from build123d import *

# Parameters (mm, degrees)
BOSS_EXTRUDE1_DEPTH = 20
BOSS_EXTRUDE2_DEPTH = 40
SKETCH1_4_W         = 15
SKETCH1_4_H         = 20
BOSS_EXTRUDE3_DEPTH = 20


with BuildPart() as part:
    # Sketch1 → Boss-Extrude1 (new body)
    with BuildSketch(Plane(origin=(0, 0, 0), x_dir=(1, 0, 0), z_dir=(0, 1, 0))):
        Polygon((20, -30), (0, -30), (0, -50), (15, -100), (22.5, -100), (22.5, -70), (35, -70), (35, -30), align=None)
        Polygon((50, -30), (35, -30), (35, -70), (47.5, -70), (47.5, -100), (55, -100), (70, -50), (70, -30), align=None)
    extrude(amount=BOSS_EXTRUDE1_DEPTH)

    # Sketch1_3 → Boss-Extrude2 (add)
    with BuildSketch(Plane(origin=(0, 0, 0), x_dir=(1, 0, 0), z_dir=(0, 1, 0))):
        Polygon((0, -30), (0, 0), (15, 0), (15, -10), (20, -10), (20, -30), align=None)
        Polygon((70, -30), (70, 0), (55, 0), (55, -10), (50, -10), (50, -30), align=None)
    extrude(amount=BOSS_EXTRUDE2_DEPTH)

    # Sketch1_4 → Boss-Extrude3 (add)
    with BuildSketch(Plane(origin=(0, 0, 0), x_dir=(1, 0, 0), z_dir=(0, 1, 0))):
        with Locations((27.5, -20)):
            Rectangle(SKETCH1_4_W, SKETCH1_4_H)
        with Locations((42.5, -20)):
            Rectangle(SKETCH1_4_W, SKETCH1_4_H)
    extrude(amount=BOSS_EXTRUDE3_DEPTH)


solid = part.part
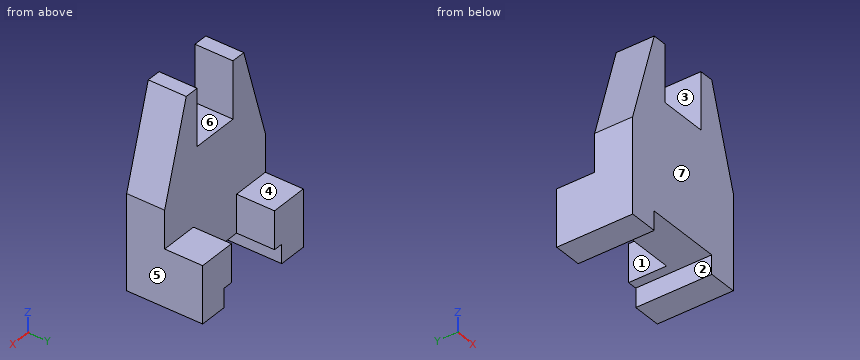
Here's how the part is built. I have some questions about the finished solid (model axes, mm). Face numbers are marked on the shaded views. A direction names the side the tool comes from. Give positions to 0.01 mm unless a question says otherwise; leave off trailing zeros. Write each loop counter-clockwise with the first axis right and the second up, starting at its lowest first coordinate (ties: lowest second). Pieces come first, ordered by that corner, then holes. Notation, with made-up numbers: (-7, 71) -> (4, 71) arc R12 cw to (4, 93) -> close; hole circle Ø1 at (17, 4.5). An arc over 180 degrees is marked (long way). Use one line per item in the form item = value. Start each with the question number.
1. Imagine slicing it at C-C on y = 4.5. List the corners of the cut face in (x, z) for me, plus the area to 3 significant figures.
2. Imagine slicing it at A-A on y = 22.5. List the corners of the cut face in (x, z) for me.
3. Thinking about a two-plate mould opening in X: for the marked faces 5, 6 and 7, which applies, +X half, -X half, draft (parallel to the pull), parting line (faces both ways), or undercut?
4. Will these pins go through, and if not, where does the flat tip stop? pin 1 Ø1 at (x, z) = (11, 40.5) entering from +Y; pin 2 Ø16 at (y, z) = (13, 83.5) entering from -X; pin 3 Ø10 at (y, z) = (6.5, 85) entering from +X.
5. If I drill on L1, parallel to Y at x = 13, z = 85.5; L2, parallel to Z at x = 6.5, y = 27; L3, parallel to X at y = 16, z = 87.5, over which ranges is the centre line in solid material (lowest first)?
6. Imagine slicing it at D-D on x = 10.5. List the corners of the cut face in (y, z) for me, plus the area to 3 significant figures.
7. On a 3-axis mill with a long thin cutter (end or side, diameter ignored), from which of +Z, -Z, +X, -X, +Y, -Y can I reach the whole of each face in a straight line? I mean the marked faces 1, 2, 3 and 4. Say none if no direction works.
8. Imagine slicing it at B-B on z = 83.5. List the corners of the cut face in (x, y) for me, plus the area to 3 significant figures.
Entries:
q1.outline = (0, 0) -> (15, 0) -> (15, 10) -> (55, 10) -> (55, 0) -> (70, 0) -> (70, 50) -> (55, 100) -> (47.5, 100) -> (47.5, 70) -> (22.5, 70) -> (22.5, 100) -> (15, 100) -> (0, 50) -> close
q1.area = 5,100 mm²
q2.outline = (0, 0) -> (15, 0) -> (15, 10) -> (20, 10) -> (20, 30) -> (0, 30) -> close; (50, 10) -> (55, 10) -> (55, 0) -> (70, 0) -> (70, 30) -> (50, 30) -> close
q3.face_5 = +X half
q3.face_6 = undercut
q3.face_7 = draft
q4.pin_1 = 20
q4.pin_2 = 7.65
q4.pin_3 = 61
q5.L1 = 0 to 20
q5.L2 = 0 to 30
q5.L3 = 11.25 to 22.5, 47.5 to 58.75
q6.outline = (0, 0) -> (40, 0) -> (40, 30) -> (20, 30) -> (20, 85) -> (0, 85) -> close
q6.area = 2,300 mm²
q7.face_1 = +Z, -Z, +Y
q7.face_2 = -Z, +Y, -Y
q7.face_3 = +Z, +Y, -Y
q7.face_4 = +Z, +X, -X, +Y
q8.outline = (10.05, 0) -> (22.5, 0) -> (22.5, 20) -> (10.05, 20) -> close; (47.5, 0) -> (59.95, 0) -> (59.95, 20) -> (47.5, 20) -> close
q8.area = 498 mm²
